Part model, mm, in its own coordinate system. Face numbers are marked on the shaded views. A direction names the side the tool comes from. Give positions to 0.01 mm unless a question says otherwise; leave off trailing zeros. Order: outer loops, then holes, each group sorted by start corner. A loop starts at its lowest first (then second) coordinate and runs counter-clockwise, first axis right, second up.
1. Which spindle directions (+Z, -Z, +X, -X, +Y, -Y) get a long thin tool onto all of the face, cutting with end or side? Do the marked faces 4 and 5. Say none if no direction does.
2. Slice it at B-B on y = 12.75. List the corners of the cut face in (x, z), and give its area (3 significant figures).
3. Slice it at A-A on z = 0. List the corners of the cut face in (x, y), and give its area (3 significant figures).
4. Drop flat-ended pins along their axis: pin 1 Ø1 at (x, z) = (5.5, -7.5) entering from +Y; pin 2 Ø1.8 at (x, z) = (1, 9.5) entering from -Y; pin 3 Ø3 at (x, z) = (0, 10.5) entering from +Y; pin 4 Ø4 at (x, y) = (3, 5) entering from +Z. Give the stop position or say it passes through.
5. Probe line 1 (X direction, y = 9, z = 0); line 2 (Y direction, x = 10.5, z = -8); line 3 (Z direction, x = 2.5, y = 2). List the from-to ranges inside material, lowest first.
6. Mould opens along Z. For the marked faces 1, 2 and 3 say: +Z half, -Z half, draft (parallel to the pull), parting line (faces both ways), or undercut.
7. Slice it at C-C on y = 1.75. List the corners of the cut face in (x, z).
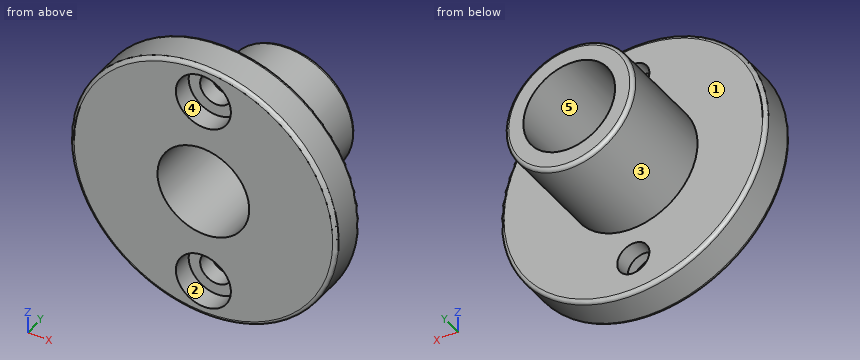
from build123d import *

# Parameters (mm, degrees)
SKETCH_1_R          = 14.5
SKETCH_1_R_2        = 7
EXTRUDE_1_DEPTH     = 4
SKETCH_1_3_R        = 7
SKETCH_1_3_R_2      = 5
EXTRUDE_2_DEPTH     = 15
SKETCH_2_R          = 3
SKETCH_2_R_2        = 1.75
CUT_EXTRUDE_1_DEPTH = 2.2
SKETCH_2_4_R        = 1.75
CUT_EXTRUDE_2_DEPTH = 26.406692032
FILLET_1_R          = 0.4


with BuildPart() as part:
    # Sketch 1 → Extrude 1 (new body)
    with BuildSketch(Plane(origin=(0, 0, 0), x_dir=(1, 0, 0), z_dir=(0, 1, 0))):
        with Locations(Location((0, 0, 0), (0, 0, 270))):
            Circle(SKETCH_1_R)
        with Locations(Location((0, 0, 0), (0, 0, 270))):
            Circle(SKETCH_1_R_2, mode=Mode.SUBTRACT)
    extrude(amount=EXTRUDE_1_DEPTH)

    # Sketch 1_3 → Extrude 2 (add)
    with BuildSketch(Plane(origin=(0, 0, 0), x_dir=(1, 0, 0), z_dir=(0, 1, 0))):
        with Locations(Location((0, 0, 0), (0, 0, 270))):
            Circle(SKETCH_1_3_R)
        with Locations(Location((0, 0, 0), (0, 0, 270))):
            Circle(SKETCH_1_3_R_2, mode=Mode.SUBTRACT)
    extrude(amount=EXTRUDE_2_DEPTH)

    # Sketch 2 → Cut-Extrude 1 (cut)
    # profile 1 of 2: a face of its own
    with BuildSketch(Plane.XZ):
        with Locations(Location((0, 10.5, 0), (0, 0, 270))):
            Circle(SKETCH_2_R)
        with Locations(Location((0, 10.5, 0), (0, 0, 270))):
            Circle(SKETCH_2_R_2, mode=Mode.SUBTRACT)
    # profile 2 of 2: a face of its own
    with BuildSketch(Plane.XZ):
        with Locations(Location((0, -10.5, 0), (0, 0, 270))):
            Circle(SKETCH_2_R)
        with Locations(Location((0, -10.5, 0), (0, 0, 270))):
            Circle(SKETCH_2_R_2, mode=Mode.SUBTRACT)
    extrude(amount=-CUT_EXTRUDE_1_DEPTH, mode=Mode.SUBTRACT)

    # Sketch 2_4 → Cut-Extrude 2 (cut, through all)
    with BuildSketch(Plane.XZ):
        with Locations(Location((0, 10.5, 0), (0, 0, 270))):
            Circle(SKETCH_2_4_R)
        with Locations(Location((0, -10.5, 0), (0, 0, 270))):
            Circle(SKETCH_2_4_R)
    extrude(amount=-CUT_EXTRUDE_2_DEPTH, mode=Mode.SUBTRACT)

    # Fillet 1
    fillet_1_edges = [part.edges().sort_by_distance(p)[0] for p in [
        (0, 4, -14.5),
        (0, 0, -14.5),
        (0, 15, -7),
    ]]
    fillet(fillet_1_edges, radius=FILLET_1_R)


solid = part.part
Data:
1. face 4: -Y
1. face 5: +Y, -Y
2. outline: circle Ø14 at (0, 0); hole circle Ø10 at (0, 0)
2. area: 75.4 mm2
3. outline: (-14.5, 0.4) arc R0.4 ccw to (-14.1, 0) - (-5, 0) - (-5, 15) - (-6.6, 15) arc R0.4 ccw to (-7, 14.6) - (-7, 4) - (-14.1, 4) arc R0.4 ccw to (-14.5, 3.6) - close; (5, 0) - (14.1, 0) arc R0.4 ccw to (14.5, 0.4) - (14.5, 3.6) arc R0.4 ccw to (14.1, 4) - (7, 4) - (7, 14.6) arc R0.4 ccw to (6.6, 15) - (5, 15) - close
3. area: 120 mm2
4. pin 1: stops at y = 4
4. pin 2: stops at y = 2.2
4. pin 3: passes through
4. pin 4: stops at z = 14.42
5. line 1: x = -7 to -5, 5 to 7
5. line 2: y = 0 to 4
5. line 3: z = -14.28 to -12.16, -8.84 to -4.33, 4.33 to 8.84, 12.16 to 14.28
6. face 1: draft
6. face 2: undercut
6. face 3: parting line
7. outline: circle Ø29 at (0, 0); hole circle Ø10 at (0, 0); hole circle Ø6 at (0, -10.5); hole circle Ø6 at (0, 10.5)
